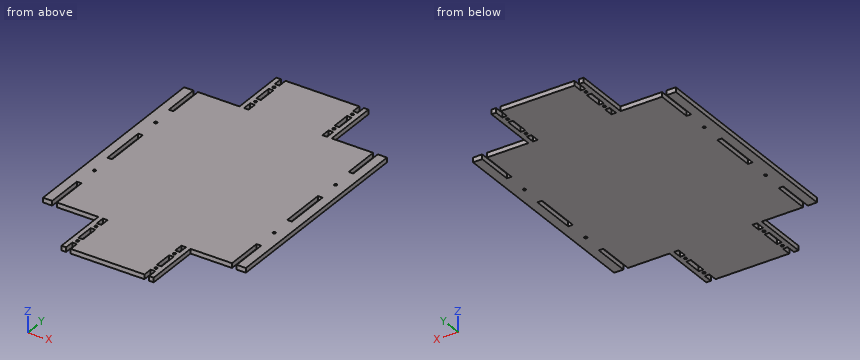
```python
from build123d import *

# Parameters (mm, degrees)
SKETCH1_W           = 220
SKETCH1_H           = 350
BOSS_EXTRUDE1_DEPTH = 5
SKETCH2_W           = 60
SKETCH2_H           = 60
CUT_EXTRUDE2_DEPTH  = 5
SKETCH3_W           = 5
SKETCH3_H           = 10
SKETCH3_H_2         = 20
CUT_EXTRUDE3_DEPTH  = 5
SKETCH4_R           = 1.5
CUT_EXTRUDE4_DEPTH  = 5
SKETCH5_W           = 5
SKETCH5_H           = 40
SKETCH5_H_2         = 50
CUT_EXTRUDE5_DEPTH  = 5
SKETCH6_R           = 1.5
CUT_EXTRUDE6_DEPTH  = 5


with BuildPart() as part:
    # Sketch1 → Boss-Extrude1 (new body)
    with BuildSketch(Plane.XY):
        Rectangle(SKETCH1_W, SKETCH1_H)
    extrude(amount=BOSS_EXTRUDE1_DEPTH)

    # Sketch2 → Cut-Extrude2 (cut)
    with BuildSketch(Plane.XY.offset(5)):
        with Locations((-80, -145)):
            Rectangle(SKETCH2_W, SKETCH2_H)
        with Locations((80, -145)):
            Rectangle(SKETCH2_W, SKETCH2_H)
        with Locations((80, 145)):
            Rectangle(SKETCH2_W, SKETCH2_H)
        with Locations((-80, 145)):
            Rectangle(SKETCH2_W, SKETCH2_H)
    extrude(amount=-CUT_EXTRUDE2_DEPTH, mode=Mode.SUBTRACT)

    # Sketch3 → Cut-Extrude3 (cut)
    with BuildSketch(Plane.XY.offset(5)):
        with Locations((42.5, 170)):
            Rectangle(SKETCH3_W, SKETCH3_H)
        with Locations((42.5, 145)):
            Rectangle(SKETCH3_W, SKETCH3_H_2)
        with Locations((42.5, 120)):
            Rectangle(SKETCH3_W, SKETCH3_H)
        with Locations((-42.5, 170)):
            Rectangle(SKETCH3_W, SKETCH3_H)
        with Locations((-42.5, 145)):
            Rectangle(SKETCH3_W, SKETCH3_H_2)
        with Locations((-42.5, 120)):
            Rectangle(SKETCH3_W, SKETCH3_H)
        with Locations((42.5, -120)):
            Rectangle(SKETCH3_W, SKETCH3_H)
        with Locations((42.5, -145)):
            Rectangle(SKETCH3_W, SKETCH3_H_2)
        with Locations((42.5, -170)):
            Rectangle(SKETCH3_W, SKETCH3_H)
        with Locations((-42.5, -120)):
            Rectangle(SKETCH3_W, SKETCH3_H)
        with Locations((-42.5, -145)):
            Rectangle(SKETCH3_W, SKETCH3_H_2)
        with Locations((-42.5, -170)):
            Rectangle(SKETCH3_W, SKETCH3_H)
    extrude(amount=-CUT_EXTRUDE3_DEPTH, mode=Mode.SUBTRACT)

    # Sketch4 → Cut-Extrude4 (cut)
    with BuildSketch(Plane.XY.offset(5)):
        with Locations((-42.5, 160)):
            Circle(SKETCH4_R)
        with Locations(Location((42.5, 160, 0), (0, 0, 180))):
            Circle(SKETCH4_R)
        with Locations((-42.5, 130)):
            Circle(SKETCH4_R)
        with Locations((42.5, 130)):
            Circle(SKETCH4_R)
        with Locations((-42.5, -160)):
            Circle(SKETCH4_R)
        with Locations((-42.5, -130)):
            Circle(SKETCH4_R)
        with Locations((42.5, -130)):
            Circle(SKETCH4_R)
        with Locations((42.5, -160)):
            Circle(SKETCH4_R)
    extrude(amount=-CUT_EXTRUDE4_DEPTH, mode=Mode.SUBTRACT)

    # Sketch5 → Cut-Extrude5 (cut)
    with BuildSketch(Plane.XY.offset(5)):
        with Locations((-97.5, -95)):
            Rectangle(SKETCH5_W, SKETCH5_H)
        with Locations((-97.5, 0)):
            Rectangle(SKETCH5_W, SKETCH5_H_2)
        with Locations((-97.5, 95)):
            Rectangle(SKETCH5_W, SKETCH5_H)
        with Locations((97.5, 95)):
            Rectangle(SKETCH5_W, SKETCH5_H)
        with Locations((97.5, 0)):
            Rectangle(SKETCH5_W, SKETCH5_H_2)
        with Locations((97.5, -95)):
            Rectangle(SKETCH5_W, SKETCH5_H)
    extrude(amount=-CUT_EXTRUDE5_DEPTH, mode=Mode.SUBTRACT)

    # Sketch6 → Cut-Extrude6 (cut)
    with BuildSketch(Plane.XY.offset(5)):
        with Locations((-97.5, 50)):
            Circle(SKETCH6_R)
        with Locations((-97.5, -50)):
            Circle(SKETCH6_R)
        with Locations((97.5, 50)):
            Circle(SKETCH6_R)
        with Locations((97.5, -50)):
            Circle(SKETCH6_R)
    extrude(amount=-CUT_EXTRUDE6_DEPTH, mode=Mode.SUBTRACT)


solid = part.part
```
Input: part model. Units: mm. Frame: model coordinates. Give positions to 0.01 mm unless a question says otherwise; leave off trailing zeros. Loops run counter-clockwise (first coordinate to the right, second up) from the corner with the lowest first, then second, coordinate; pieces in that order, holes last.
1) Section query C-C on z = 0.8. Count the separate pieces of the cut face and the enclosed holes in it, and give its area (3 significant figures).
A:
separate pieces: 1
enclosed holes: 22
area: 60,400 mm2
2) Contact query for flat-ended pins moving along their axis: pin 1 (2.5 mm diameter, centred on x = -76, z = 2.5, fed in from +Y); pin 2 (2.5 mm diameter, centred on x = 82, z = 1.5, fed in from -Y); pin 3 (2.5 mm diameter, centred on y = -170.5, z = 3, fed in from +X). Output: stop coordinate, or through.
A:
pin 1: stops at y = 115
pin 2: stops at y = -115
pin 3: stops at x = 50
3) Section query B-B on x = 58. Return the cut outline in (y, z).
A:
outline: (-115, 0) - (115, 0) - (115, 5) - (-115, 5) - close
4) Line query: L1, parallel to X at y = 160, z = 2.6; L2, parallel to X at y = 110, z = 2; L3, parallel to Y at x = -44.5, z = 2.65. Output: solid intervals per line, ascending.
A:
L1: x = -50 to -44, -41 to 41, 44 to 50
L2: x = -110 to -100, -95 to 95, 100 to 110
L3: y = -165 to -155, -135 to -125, -115 to 115, 125 to 135, 155 to 165
5) Section query A-A on y = -85. Return the cut outline in (x, z), and give its area (3 significant figures).
A:
outline: (-110, 0) - (-100, 0) - (-100, 5) - (-110, 5) - close; (-95, 0) - (95, 0) - (95, 5) - (-95, 5) - close; (100, 0) - (110, 0) - (110, 5) - (100, 5) - close
area: 1,050 mm2
